from build123d import *

# Parameters (mm, degrees)
SKETCH1_R      = 2.35
SKETCH1_W      = 15
SKETCH1_H      = 3.1
EXTRUDE1_DEPTH = 3.1


with BuildPart() as part:
    # Sketch1 → Extrude1 (new body)
    with BuildSketch(Plane.XY):
        Polygon((-41.013157114, 34.508489293), (-10.513157114, 34.508489293), (-10.513157114, 32.508489293), (-18.263157114, 32.508489293), (-18.263157114, 29.408489293), (-10.513157114, 29.408489293), (-10.513157114, 7.058489293), (-41.013157114, 7.058489293), (-41.013157114, 29.408489293), (-33.263157114, 29.408489293), (-33.263157114, 32.508489293), (-41.013157114, 32.508489293), align=None)
        with Locations(Location((-14.388157114, 26.058489293, 0), (0, 0, 180))):
            Circle(SKETCH1_R, mode=Mode.SUBTRACT)
        with Locations(Location((-37.138157114, 26.058489293, 0), (0, 0, 180))):
            Circle(SKETCH1_R, mode=Mode.SUBTRACT)
        with Locations(Location((-25.763157114, 15.508489293, 0), (0, 0, 180))):
            Circle(SKETCH1_R, mode=Mode.SUBTRACT)
        with BuildLine():
            Line((-37.138157114, 21.287155622), (-37.138157114, 14.158489293))
            ThreePointArc((-37.138157114, 14.158489293), (-36.845263895, 13.451382512), (-36.138157114, 13.158489293))
            Line((-36.138157114, 13.158489293), (-33.725119975, 13.158489293))
            ThreePointArc((-33.725119975, 13.158489293), (-33.328320215, 13.240584097), (-32.996670851, 13.473389392))
            Line((-32.996670851, 13.473389392), (-28.585897467, 18.16325141))
            ThreePointArc((-28.585897467, 18.16325141), (-25.763157114, 19.383489293), (-22.940416761, 18.16325141))
            Line((-22.940416761, 18.16325141), (-18.529643377, 13.473389392))
            ThreePointArc((-18.529643377, 13.473389392), (-18.197994013, 13.240584097), (-17.801194253, 13.158489293))
            Line((-17.801194253, 13.158489293), (-15.388157114, 13.158489293))
            ThreePointArc((-15.388157114, 13.158489293), (-14.681050333, 13.451382512), (-14.388157114, 14.158489293))
            Line((-14.388157114, 14.158489293), (-14.388157114, 21.287155622))
            ThreePointArc((-14.388157114, 21.287155622), (-14.611907088, 21.917580794), (-15.183028909, 22.265890734))
            ThreePointArc((-15.183028909, 22.265890734), (-17.128195891, 23.318450516), (-18.180755673, 25.263617499))
            ThreePointArc((-18.180755673, 25.263617499), (-18.529065613, 25.834739319), (-19.159490785, 26.058489293))
            Line((-19.159490785, 26.058489293), (-32.366823443, 26.058489293))
            ThreePointArc((-32.366823443, 26.058489293), (-32.997248615, 25.834739319), (-33.345558555, 25.263617499))
            ThreePointArc((-33.345558555, 25.263617499), (-34.398118337, 23.318450516), (-36.343285319, 22.265890734))
            ThreePointArc((-36.343285319, 22.265890734), (-36.91440714, 21.917580794), (-37.138157114, 21.287155622))
        make_face(mode=Mode.SUBTRACT)
        with Locations((-25.763157114, 10.608489293)):
            Rectangle(SKETCH1_W, SKETCH1_H, mode=Mode.SUBTRACT)
    extrude(amount=EXTRUDE1_DEPTH)


solid = part.part
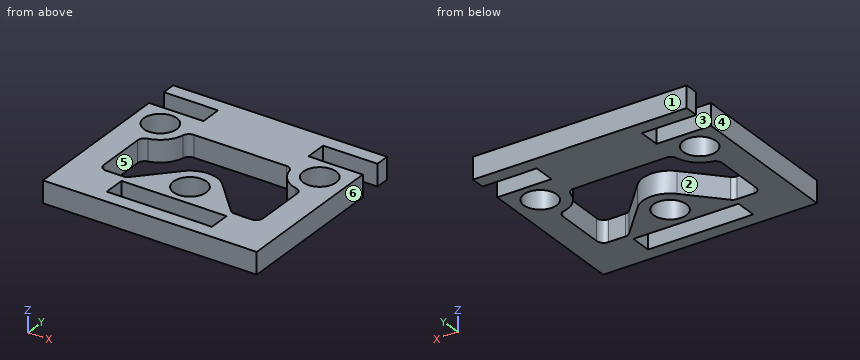
Verification items for the finished model (mm, model axes). Face numbers are marked on the shaded views. A direction names the side the tool comes from. Coordinates: 2 decimals unless noted, no trailing zeros. Order: outer loops, then holes, each group sorted by start corner. A loop starts at its lowest first (then second) coordinate and runs counter-clockwise, first axis right, second up. Notation, with made-up numbers: M 78,-21.75 L 95,-21.75 A20 cw 95,13.25 Z; hole C -9.75,8.5 d10. An arc over 180 degrees is marked long. One line per item, written item: value. Start each with the question number.
Item 1: Sectioned sample at B-B (x = -21). Enter the section's corners in (y, z).
Item 2: Mould release check, pull along X, two halves, no side actions. Record for the marked faces 3, 4, 5 and 6: released by +X, released by -X, zero draft, split by the parting line, or undercut.
Item 3: Access from +Z, -Z, +X, -X, +Y, -Y to the whole of each face (thin tool, end or side, straight path). Record for the marked faces 1 and 2.
Item 4: Sectioned sample at D-D (y = 30.75). Enter the section's corners in (x, z).
Item 5: Sectioned sample at C-C (x = -26.5). Enter the section's corners in (y, z), then the cut area to 3 significant figures.
Item 6: Sectioned sample at A-A (y = 16.5). Enter the section's corners in (x, z), then the cut area to 3 significant figures.
Item 7: Scan lines: probe 1 along X at (y, z) = (10, 1.4); probe 2 along Y at (x, z) = (-14, 0.6); probe 3 along X at (y, z) = (24.5, 1.55). Record each from-to range of solid material in increasing order.
Item 8: Gauge pin test, flat ends, axial feed: pin 1 (0.9 mm diameter, centred on y = 30.5, z = 2, fed in from -X); pin 2 (0.9 mm diameter, centred on y = 31, z = 2, fed in from +X); pin 3 (10 mm diameter, centred on x = -27.5, y = 21, fed in from -Z). Record the tip position at first contact, or that the pin passes through.
Conclusion:
1. outline: M 7.06,0 L 9.06,0 L 9.06,3.1 L 7.06,3.1 Z; M 12.16,0 L 16.1,0 L 16.1,3.1 L 12.16,3.1 Z; M 26.06,0 L 34.51,0 L 34.51,3.1 L 26.06,3.1 Z
2. face 3: zero draft
2. face 4: released by -X
2. face 5: undercut
2. face 6: released by +X
3. face 1: +Z, -Z, +X, -X, +Y
3. face 2: +Z, -Z
4. outline: M -33.26,0 L -18.26,0 L -18.26,3.1 L -33.26,3.1 Z
5. outline: M 7.06,0 L 9.06,0 L 9.06,3.1 L 7.06,3.1 Z; M 12.16,0 L 13.28,0 L 13.28,3.1 L 12.16,3.1 Z; M 17.74,0 L 19.31,0 L 19.31,3.1 L 17.74,3.1 Z; M 26.06,0 L 34.51,0 L 34.51,3.1 L 26.06,3.1 Z
5. area: 40.7 mm^2
6. outline: M -41.01,0 L -37.14,0 L -37.14,3.1 L -41.01,3.1 Z; M -30.15,0 L -27.89,0 L -27.89,3.1 L -30.15,3.1 Z; M -23.63,0 L -21.38,0 L -21.38,3.1 L -23.63,3.1 Z; M -14.39,0 L -10.51,0 L -10.51,3.1 L -14.39,3.1 Z
6. area: 38.0 mm^2
7. probe 1: x = -41.01 to -33.26, -18.26 to -10.51
7. probe 2: y = 7.06 to 23.74, 28.38 to 29.41, 32.51 to 34.51
7. probe 3: x = -41.01 to -38.9, -35.38 to -33.59, -17.94 to -16.15, -12.63 to -10.51
8. pin 1: stops at x = -33.26
8. pin 2: stops at x = -18.26
8. pin 3: stops at z = 0
